```python
from build123d import *

# Parameters (mm, degrees)
SKETCH_R     = 7.5
PAD_DEPTH    = 30
SKETCH001_W  = 17.539976
SKETCH001_H  = 16.208446
PAD001_DEPTH = 3


with BuildPart() as part:
    # Sketch → Pad (new body)
    with BuildSketch(Plane.XY):
        Circle(SKETCH_R)
    extrude(amount=PAD_DEPTH)

    # Sketch001 → Pad001 (join)
    with BuildSketch(Plane.XY.offset(30)):
        Rectangle(SKETCH001_W, SKETCH001_H)
    extrude(amount=PAD001_DEPTH)


solid = part.part
```
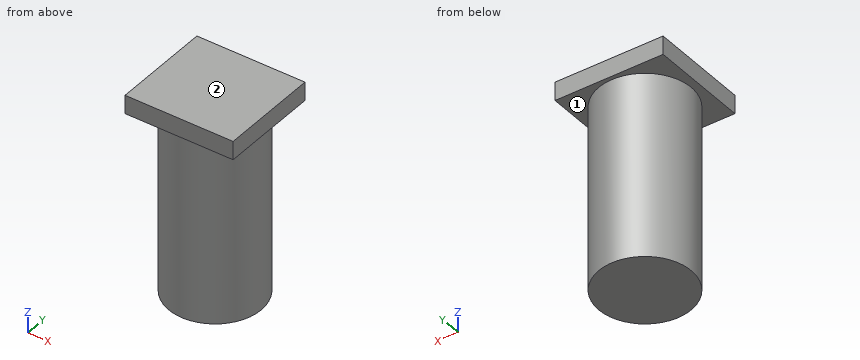
The model under review builds one solid part; all positions refer to its coordinate system, in mm. Face numbers are marked on the shaded views. A direction names the side the tool comes from. Give positions to 0.01 mm unless a question says otherwise; leave off trailing zeros. Write each loop counter-clockwise with the first axis right and the second up, starting at its lowest first coordinate (ties: lowest second). Pieces come first, ordered by that corner, then holes. Notation, with made-up numbers: M 78,-35.5 L 86,-35.5 A19 ccw 86,-3.5 Z; hole C -5.75,68.25 d2. An arc over 180 degrees is marked long. Write each question's results on one line, items separated by ' | '. Start each with the question number.
1. We need section B-B (y = 0). Write out the cut boundary in (x, z), and give its area (3 significant figures).
2. Insertion check: pin 1 Ø1.5 at (y, z) = (6, 15) entering from -X; pin 2 Ø2 at (y, z) = (-4.5, 27.5) entering from +X; pin 3 Ø5 at (x, z) = (-2.5, 5) entering from -Y; pin 4 Ø4 at (y, z) = (2, 28.5) entering from -X. Each pin has a flat end and moves straight along its axis. Give the tip position at first contact, or say it passes through.
3. For the marked faces 1 and 2, list the 3-axis set-ups (+Z, -Z, +X, -X, +Y, -Y) from which the entire face can be reached by the end or side of a thin tool; tool diameter is ignored.
4. For probe 1 along Z at (x, y) = (5.25, -6.5); probe 2 along X at (y, z) = (0.25, 26); probe 3 along Y at (x, z) = (-4.5, 9.5), list the stretches that pass through material, from the lowest coordinate up. Write a range as [from, to].
5. We need section C-C (z = 13.5). Write out the cut boundary in (x, y), and give its area (3 significant figures).
6. We need section A-A (x = -4.5). Write out the cut boundary in (y, z), and give its area (3 significant figures).
Results found:
1) outline: M -8.77,30 L -7.5,30 L -7.5,0 L 7.5,0 L 7.5,30 L 8.77,30 L 8.77,33 L -8.77,33 Z | area: 503 mm^2
2) pin 1: stops at x = -5.36 | pin 2: stops at x = 6.63 | pin 3: stops at y = -7.5 | pin 4: stops at x = -8.77
3) face 1: -Z | face 2: +Z, +X, -X, +Y, -Y
4) probe 1: z = [30, 33] | probe 2: x = [-7.5, 7.5] | probe 3: y = [-6, 6]
5) outline: C 0,0 d15 | area: 177 mm^2
6) outline: M -8.1,30 L -6,30 L -6,0 L 6,0 L 6,30 L 8.1,30 L 8.1,33 L -8.1,33 Z | area: 409 mm^2
